Source: three-view drawing plus pictorial views. Frame: mm from the lowest corner of the part. A direction names the side the tool comes from. Give positions to 0.01 mm unless a question says otherwise; leave off trailing zeros. Loops run counter-clockwise (first coordinate to the right, second up) from the corner with the lowest first, then second, coordinate; pieces in that order, holes last. Notation, with made-up numbers: (45, 21) - (78, 21) arc R36 ccw to (78, 56) - close; hole circle Ø2 at (13.5, 82). An arc over 180 degrees is marked (long way). Answer in a Markdown table with one row per item.
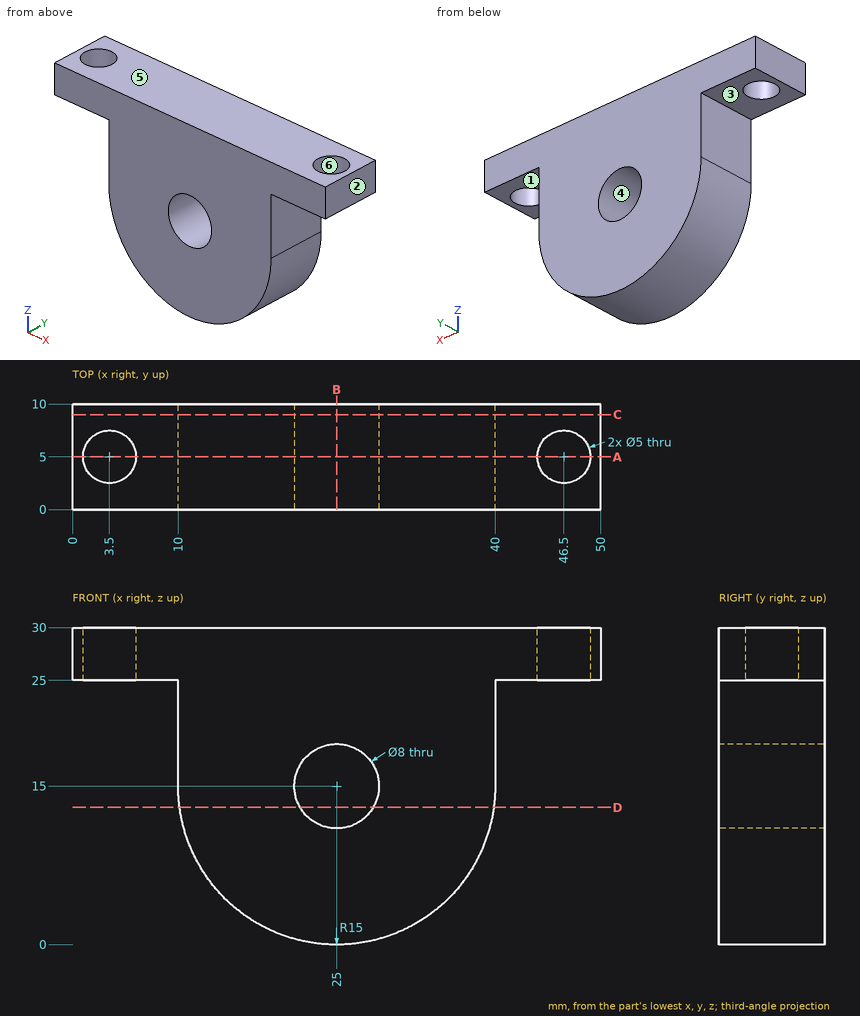
Q1. Cut plane A-A (y = 5). Output: boundary loops of the cut face in (x, z), and give its area (3 significant figures).
Check values:
| item | result |
|---|---|
| outline | (0, 25) - (1, 25) - (1, 30) - (0, 30) - close; (6, 25) - (10, 25) - (10, 15) arc R15 ccw to (40, 15) - (40, 25) - (44, 25) - (44, 30) - (6, 30) - close; (49, 25) - (50, 25) - (50, 30) - (49, 30) - close; hole circle Ø8 at (25, 15) |
| area | 803 mm² |
Q2. Draft query along Z for the marked faces 4, 5 and 6. Return one class per face: pulls with the +Z half, pulls with the -Z half, needs draft (parallel to the pull), parting line crosses it, or undercut.
Check values:
| item | result |
|---|---|
| face 4 | undercut |
| face 5 | pulls with the +Z half |
| face 6 | needs draft |
Q3. Reachability of the marked faces 1, 2 and 3 from +Z, -Z, +X, -X, +Y, -Y: full face, straight path, thin tool, end or side. Return the list, or none.
Check values:
| item | result |
|---|---|
| face 1 | -Z, +X, +Y, -Y |
| face 2 | +Z, -Z, +X, +Y, -Y |
| face 3 | -Z, -X, +Y, -Y |
Q4. Cut plane C-C (y = 9). Output: boundary loops of the cut face in (x, z), and give its area (3 significant figures).
Check values:
| item | result |
|---|---|
| outline | (0, 25) - (10, 25) - (10, 15) arc R15 ccw to (40, 15) - (40, 25) - (50, 25) - (50, 30) - (0, 30) - close; hole circle Ø8 at (25, 15) |
| area | 853 mm² |
Q5. Cut plane D-D (z = 13). Output: boundary loops of the cut face in (x, y), and give its area (3 significant figures).
Check values:
| item | result |
|---|---|
| outline | (10.13, 0) - (21.54, 0) - (21.54, 10) - (10.13, 10) - close; (28.46, 0) - (39.87, 0) - (39.87, 10) - (28.46, 10) - close |
| area | 228 mm² |
Q6. First-contact query: pin 1 (5 mm diameter, centred on y = 6, z = 20, fed in from +X); pin 2 (1 mm diameter, centred on x = 32, y = 1.5, fed in from -Z); pin 3 (3 mm diameter, centred on y = 6.5, z = 22, fed in from -X); pin 4 (10 mm diameter, centred on x = 44.5, z = 23, fed in from -Y). Flat tips, straight axial feed; report the tip coordinate or a pass-through.
Check values:
| item | result |
|---|---|
| pin 1 | x = 40 |
| pin 2 | z = 1.48 |
| pin 3 | x = 10 |
| pin 4 | y = 0 |
Q7. Material intervals for line 1 along X through (y, z) = (3.25, 15); line 2 along Y through (x, z) = (3.5, 28.75); line 3 along Z through (x, y) = (13, 1.5), sorted ascending.
Check values:
| item | result |
|---|---|
| line 1 | 10 to 21, 29 to 40 |
| line 2 | 0 to 2.5, 7.5 to 10 |
| line 3 | 6 to 30 |
Q8. Cut plane B-B (x = 25). Output: boundary loops of the cut face in (y, z), and give its area (3 significant figures).
Check values:
| item | result |
|---|---|
| outline | (0, 0) - (10, 0) - (10, 11) - (0, 11) - close; (0, 19) - (10, 19) - (10, 30) - (0, 30) - close |
| area | 220 mm² |
